from build123d import *

# Parameters (mm, degrees)
SKETCH1_R           = 4
SKETCH1_R_2         = 7.5
BOSS_EXTRUDE1_DEPTH = 10
SKETCH2_R           = 7.5
SKETCH2_R_2         = 6
BOSS_EXTRUDE2_DEPTH = 6
CUT_EXTRUDE2_DEPTH  = 6
SKETCH4_R           = 12.5
CUT_EXTRUDE1_DEPTH  = 16
SKETCH8_W           = 7.25
SKETCH8_H           = 20
SKETCH8_R           = 1.2
BOSS_EXTRUDE3_DEPTH = 15
SKETCH10_W          = 15.5
SKETCH10_H          = 1
BOSS_EXTRUDE4_DEPTH = 15
FILLET1_R           = 1.5
CHAMFER1_SIZE       = 2.5


with BuildPart() as part:
    # Sketch1 → Boss-Extrude1 (new, symmetric)
    with BuildSketch(Plane.XY):
        with BuildLine():
            Line((-15, -80), (-15, 20))
            Line((-15, 20), (15, 20))
            Line((15, 20), (15, -80))
            ThreePointArc((15, -80), (0, -95), (-15, -80))
        make_face()
        Circle(SKETCH1_R, mode=Mode.SUBTRACT)
        with Locations((0, -83)):
            Circle(SKETCH1_R_2, mode=Mode.SUBTRACT)
    extrude(amount=BOSS_EXTRUDE1_DEPTH, both=True)

    # Sketch2 → Boss-Extrude2 (add, symmetric)
    with BuildSketch(Plane.XY):
        with Locations((0, -83)):
            Circle(SKETCH2_R)
        with Locations((0, -83)):
            Circle(SKETCH2_R_2, mode=Mode.SUBTRACT)
    extrude(amount=BOSS_EXTRUDE2_DEPTH, both=True)

    # Sketch11 → Cut-Extrude2 (cut)
    with BuildSketch(Plane(origin=(0, 0, -10), x_dir=(-1, 0, 0), z_dir=(0, 0, -1))):
        Polygon((0, 6), (-5.196152423, 3), (-5.196152423, -3), (0, -6), (5.196152423, -3), (5.196152423, 3), align=None)
    extrude(amount=-CUT_EXTRUDE2_DEPTH, mode=Mode.SUBTRACT)

    # Sketch4 → Cut-Extrude1 (cut)
    with BuildSketch(Plane(origin=(0, 0, 10), x_dir=(-1, 0, 0), z_dir=(0, 0, -1))):
        Circle(SKETCH4_R)
    extrude(amount=CUT_EXTRUDE1_DEPTH, mode=Mode.SUBTRACT)

    # Sketch8 → Boss-Extrude3 (add)
    # profile 1 of 2: a face of its own
    with BuildSketch(Plane(origin=(0, 20, 0), x_dir=(1, 0, 0), z_dir=(0, 1, 0))):
        with Locations((-11.375, 0)):
            Rectangle(SKETCH8_W, SKETCH8_H)
        with Locations(Location((-10, -7.75, 0), (0, 0, 270))):
            Circle(SKETCH8_R, mode=Mode.SUBTRACT)
        with Locations(Location((-10, 7.75, 0), (0, 0, 90))):
            Circle(SKETCH8_R, mode=Mode.SUBTRACT)
    # profile 2 of 2: a face of its own
    with BuildSketch(Plane(origin=(0, 20, 0), x_dir=(1, 0, 0), z_dir=(0, 1, 0))):
        with Locations((11.375, 0)):
            Rectangle(SKETCH8_W, SKETCH8_H)
        with Locations(Location((10, -7.75, 0), (0, 0, 90))):
            Circle(SKETCH8_R, mode=Mode.SUBTRACT)
        with Locations(Location((10, 7.75, 0), (0, 0, 270))):
            Circle(SKETCH8_R, mode=Mode.SUBTRACT)
    extrude(amount=BOSS_EXTRUDE3_DEPTH)

    # Sketch10 → Boss-Extrude4 (add)
    with BuildSketch(Plane(origin=(0, 20, 0), x_dir=(1, 0, 0), z_dir=(0, 1, 0))):
        with Locations((0, 9.5)):
            Rectangle(SKETCH10_W, SKETCH10_H)
    extrude(amount=BOSS_EXTRUDE4_DEPTH)

    # Fillet1
    fillet1_edges = [part.edges().sort_by_distance(p)[0] for p in [
        (-7.75, 27.5, -9),
        (7.75, 27.5, -9),
        (-7.75, 27.5, 10),
        (7.75, 27.5, 10),
    ]]
    fillet(fillet1_edges, radius=FILLET1_R)

    # Chamfer1
    chamfer1_edges = [part.edges().sort_by_distance(p)[0] for p in [
        (-15, -22.5, 10),
        (0, -95, 10),
        (15, -22.5, 10),
        (15, -22.5, -10),
        (0, -95, -10),
        (-15, -22.5, -10),
    ]]
    chamfer(chamfer1_edges, length=CHAMFER1_SIZE - 0.0001)  # a hair under: the kernel refuses the full size


solid = part.part
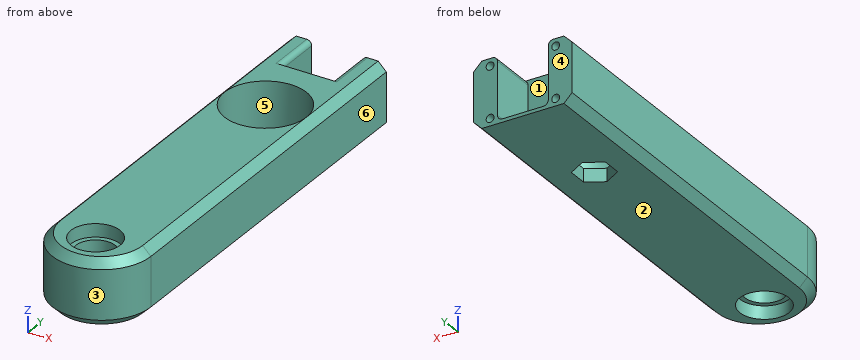
Can you work these out from the model? Positions are in its coordinate system, mm. Face numbers are marked on the shaded views. A direction names the side the tool comes from. Round coordinates to 2 decimals unless told otherwise and drop trailing zeros. Loops run counter-clockwise (first coordinate to the right, second up) from the corner with the lowest first, then second, coordinate; pieces in that order, holes last. Notation, with made-up numbers: (12.5, -30.75) - (44.5, -30.75) arc R14 cw to (44.5, -21.75) - close; hole circle Ø1 at (9.5, 37.25). An arc over 180 degrees is marked (long way). Answer in a Markdown table with one row per item. Add a question column.
Q1. I want a section at B-B on y = -62.5. List the corners of the cut face in (x, z) for me, and give its area (4 significant figures).
Q2. I need wall thicknesses on L1, parallel to Y at x = 0, z = -1.75; L2, parallel to X at y = 26.5, z = -2.25; L3, parallel to Y at x = 4.5, z = -7.5. Which ranges of each line are inside material? Lowest first, please.
Q3. Which directions (+Z, -Z, +X, -X, +Y, -Y) give clear straight access to the entire face, cutting with the end or side of a thin tool? Please do the marked faces 1 and 2.
Q4. I want a section at A-A on z = 1.75. List the corners of the cut face in (x, y) for me, and give its area (3 significant figures).
Q5. We'd pull the mould along Y, two halves only. Please class the marked faces 3, 4, 5 and 6: pulls with the +Y half, pulls with the -Y half, needs draft (parallel to the pull), parting line crosses it, or undercut.
Q6. I want a section at D-D on y = 11. List the corners of the cut face in (x, z) for me.
Q7. I want a section at C-C on x = -1.75. Count the separate pieces of the cut face and the enclosed holes in it, and give its area (3 significant figures).
Q8. For pin 1 Ø9 at (x, z) = (-0.5, 3) entering from +Y; pin 2 Ø12 at (x, z) = (8.5, -5) entering from -Y; pin 3 Ø1.4 at (x, z) = (-10, -7.75) entering from -Y, each with a flat end and sliding along its axis, tell me the tip position at first contact or that it passes through.
A:
| question | item | result |
|---|---|---|
| 1 | outline | (-15, -7.5) - (-12.5, -10) - (12.5, -10) - (15, -7.5) - (15, 7.5) - (12.5, 10) - (-12.5, 10) - (-15, 7.5) - close |
| 1 | area | 587.5 mm^2 |
| 2 | L1 | -95 to -89, -77 to -12.5, 12.5 to 20 |
| 2 | L2 | -15 to -7.75, 7.75 to 15 |
| 2 | L3 | -94.31 to -89, -77 to -3.4, 3.4 to 20 |
| 3 | face 1 | +Z, +Y |
| 3 | face 2 | -Z, +X, -X, +Y, -Y |
| 4 | outline | (-15, -80) arc R15 ccw to (15, -80) - (15, 35) - (7.75, 35) - (7.75, 20) - (-7.75, 20) - (-7.75, 35) - (-15, 35) - close; hole circle Ø25 at (0, 0); hole circle Ø12 at (0, -83) |
| 4 | area | 2,970 mm^2 |
| 5 | face 3 | pulls with the -Y half |
| 5 | face 4 | pulls with the +Y half |
| 5 | face 5 | undercut |
| 5 | face 6 | needs draft |
| 6 | outline | (-15, -7.5) - (-12.5, -10) - (12.5, -10) - (15, -7.5) - (15, 7.5) - (12.5, 10) - (5.94, 10) - (5.94, -6) - (-5.94, -6) - (-5.94, 10) - (-12.5, 10) - (-15, 7.5) - close |
| 7 | separate pieces | 3 |
| 7 | enclosed holes | 0 |
| 7 | area | 1,620 mm^2 |
| 8 | pin 1 | y = 20 |
| 8 | pin 2 | y = -94.79 |
| 8 | pin 3 | y = -91.73 |
